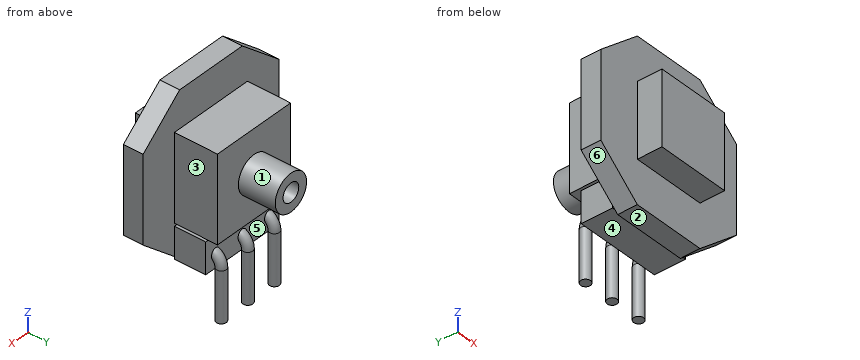
from build123d import *

# Parameters (mm, degrees)
EXTRUDE_362_DEPTH          = 1.6
SKETCH_2_W                 = 7
SKETCH_2_H                 = 7
EXTRUDE_2_DEPTH            = 3.5
SKETCH_3_R                 = 1.5
SKETCH_3_R_2               = 0.75
EXTRUDE_3_DEPTH            = 3
SKETCH_6_W                 = 6
SKETCH_6_H                 = 6
EXTRUDE_6_DEPTH            = 2
SKETCH_4_R                 = 0.4
PATTERN_LINEAR_1_COUNT     = 2
PATTERN_LINEAR_1_PITCH     = 2.54
PATTERN_LINEAR_1_COL_COUNT = 2
PATTERN_LINEAR_1_COL_PITCH = 2.54
SKETCH_8_W                 = 7
SKETCH_8_H                 = 2.54
EXTRUDE_7_DEPTH            = 2.54


with BuildPart() as part:
    # Эскиз1 → Extrude 362 (new body)
    with BuildSketch(Plane(origin=(0, 0, 0), x_dir=(1, 0, 0), z_dir=(0, 1, 0))):
        Polygon((-3, 6.5), (3, 6.5), (6.5, 3.5), (6.5, -3.5), (3, -6.5), (-3, -6.5), (-6.5, -3.5), (-6.5, 3.5), align=None)
    extrude(amount=EXTRUDE_362_DEPTH)

    # Эскиз2 → Бобышка-Вытянуть2 (add)
    with BuildSketch(Plane(origin=(0, 1.6, 0), x_dir=(1, 0, 0), z_dir=(0, 1, 0))):
        Rectangle(SKETCH_2_W, SKETCH_2_H)
    extrude(amount=EXTRUDE_2_DEPTH)

    # Эскиз3 → Бобышка-Вытянуть3 (add)
    with BuildSketch(Plane(origin=(0, 5.1, 0), x_dir=(1, 0, 0), z_dir=(0, 1, 0))):
        with Locations(Location((0, 0, 0), (0, 0, 270))):
            Circle(SKETCH_3_R)
        with Locations(Location((0, 0, 0), (0, 0, 270))):
            Circle(SKETCH_3_R_2, mode=Mode.SUBTRACT)
    extrude(amount=EXTRUDE_3_DEPTH)

    # Эскиз6 → Бобышка-Вытянуть6 (add)
    with BuildSketch(Plane.XZ):
        Rectangle(SKETCH_6_W, SKETCH_6_H)
    extrude(amount=EXTRUDE_6_DEPTH)

    # По траектории1: sweep along a path in Эскиз7
    with BuildLine(Plane(origin=(0, 0, 0), x_dir=(0, 0, -1), z_dir=(1, 0, 0))) as sweep_1_path:
        Line((5, 1.6), (5, 3.6))
        ThreePointArc((5, 3.6), (5.292893219, 4.307106781), (6, 4.6))
        Line((6, 4.6), (10.08, 4.6))
    # Эскиз4 → По траектории1 (sweep)
    with BuildSketch(Plane.XZ.offset(-1.6)):
        with Locations((0, -5)):
            Circle(SKETCH_4_R)
    sweep_1 = sweep(path=sweep_1_path.line)

    # Линейный массив1: По траектории1 ×2
    with Locations(*[(i * PATTERN_LINEAR_1_PITCH, 0, 0) for i in range(1, PATTERN_LINEAR_1_COUNT)]):
        add(sweep_1)

    # Линейный массив1 col: По траектории1 ×2
    with Locations(*[(-i * PATTERN_LINEAR_1_COL_PITCH, 0, 0) for i in range(1, PATTERN_LINEAR_1_COL_COUNT)]):
        add(sweep_1)

    # Эскиз8 → Бобышка-Вытянуть7 (add)
    with BuildSketch(Plane(origin=(0, 1.6, 0), x_dir=(1, 0, 0), z_dir=(0, 1, 0))):
        with Locations((0, 5)):
            Rectangle(SKETCH_8_W, SKETCH_8_H)
    extrude(amount=EXTRUDE_7_DEPTH)


solid = part.part
Verification items for the finished model (mm, model axes). Face numbers are marked on the shaded views. A direction names the side the tool comes from. Round coordinates to 2 decimals unless told otherwise and drop trailing zeros. Loops run counter-clockwise (first coordinate to the right, second up) from the corner with the lowest first, then second, coordinate; pieces in that order, holes last. Notation, with made-up numbers: (11, 71.5) - (18, 71.5) arc R25 ccw to (18, 94.5) - close; hole circle Ø7 at (-19.75, 79.5). An arc over 180 degrees is marked (long way). Answer in a Markdown table with one row per item. Add a question column.
Q1. Release check for a two-part mould opening along X. For the marked faces 4, 5 and 6 record: pulls with the +X half, pulls with the -X half, needs draft (parallel to the pull), parting line crosses it, or undercut.
Q2. Section check D-D on y = 4.6. State how many separate pieces and enclosed holes the cut face has, plus the area to 3 significant figures.
Q3. Gauge pin test, flat ends, axial feed: pin 1 (1 mm diameter, centred on y = -1.5, z = -1, fed in from +X); pin 2 (1 mm diameter, centred on y = 4, z = -1, fed in from -X); pin 3 (1.3 mm diameter, centred on x = 0.5, y = 1, fed in from -Z). Record the tip position at first contact, or that the pin passes through.
Q4. Section check A-A on y = 2.25. Enter the section's corners in (x, z).
Q5. Section check B-B on y = 0.25. Enter the section's corners in (x, z), plus the area to 3 significant figures.
Q6. Section check C-C on z = 0. Enter the section's corners in (x, y), plus the area to 3 significant figures.
Q7. Material ranges on line 1 (X direction, y = 7.3, z = 0); line 2 (Z direction, x = -0.75, y = 2.25); line 3 (Y direction, x = 1, z = 1.5), recorded low to high.
Q8. Tool access check on the marked faces 1, 2 and 3. Record the directions out of +Z, -Z, +X, -X, +Y, -Y that give a thin tool (end or side, any length) a straight path to the whole face; none if there is none.
Found:
| question | item | result |
|---|---|---|
| 1 | face 4 | needs draft |
| 1 | face 5 | undercut |
| 1 | face 6 | pulls with the -X half |
| 2 | separate pieces | 4 |
| 2 | enclosed holes | 0 |
| 2 | area | 60.8 mm² |
| 3 | pin 1 | stops at x = 3 |
| 3 | pin 2 | stops at x = -3.5 |
| 3 | pin 3 | stops at z = -6.5 |
| 4 | outline | (-3.5, -6.27) - (3.5, -6.27) - (3.5, -3.73) - (-3.5, -3.73) - close; (-3.5, -3.5) - (3.5, -3.5) - (3.5, 3.5) - (-3.5, 3.5) - close |
| 5 | outline | (-6.5, -3.5) - (-3, -6.5) - (3, -6.5) - (6.5, -3.5) - (6.5, 3.5) - (3, 6.5) - (-3, 6.5) - (-6.5, 3.5) - close |
| 5 | area | 148 mm² |
| 6 | outline | (-6.5, 0) - (-3, 0) - (-3, -2) - (3, -2) - (3, 0) - (6.5, 0) - (6.5, 1.6) - (3.5, 1.6) - (3.5, 5.1) - (1.5, 5.1) - (1.5, 8.1) - (0.75, 8.1) - (0.75, 5.1) - (-0.75, 5.1) - (-0.75, 8.1) - (-1.5, 8.1) - (-1.5, 5.1) - (-3.5, 5.1) - (-3.5, 1.6) - (-6.5, 1.6) - close |
| 6 | area | 61.8 mm² |
| 7 | line 1 | x = -1.5 to -0.75, 0.75 to 1.5 |
| 7 | line 2 | z = -6.27 to -3.73, -3.5 to 3.5 |
| 7 | line 3 | y = -2 to 5.1 |
| 8 | face 1 | +Y |
| 8 | face 2 | -Z, +X, -X, -Y |
| 8 | face 3 | +Z, -Z, +X, +Y |
